```python
from build123d import *

# Parameters (mm, degrees)
F0_R     = 127
F1_DEPTH = 127


with BuildPart() as f1:
    # F0 (on Front) → F1 (new body)
    with BuildSketch(Plane.XZ):
        with BuildLine():
            ThreePointArc((-317.5, 641.227615), (0, 323.727615), (317.5, 641.227615))
            ThreePointArc((317.5, 641.227615), (0, 958.727615), (-317.5, 641.227615))
        make_face()
        with Locations((0, 641.227615)):
            Circle(F0_R, mode=Mode.SUBTRACT)
        with BuildLine():
            Line((317.5, -501.772385), (317.5, 641.227615))
            ThreePointArc((317.5, 641.227615), (0, 323.727615), (-317.5, 641.227615))
            Line((-317.5, 641.227615), (-317.5, -501.772385))
            Line((-317.5, -501.772385), (317.5, -501.772385))
        make_face()
    extrude(amount=F1_DEPTH)


solid = f1.part
```
Design review of the part built by this model. Coordinates are the model's own, in mm. Round coordinates to 2 decimals unless told otherwise and drop trailing zeros. Write each loop counter-clockwise with the first axis right and the second up, starting at its lowest first coordinate (ties: lowest second). Pieces come first, ordered by that corner, then holes. Notation, with made-up numbers: (29.5, 37.25) -> (82.5, 37.25) arc R19 cw to (82.5, 67.25) -> close; hole circle Ø10 at (-20, 8). An arc over 180 degrees is marked (long way). Write item = value, one per line. Start each with the question number.
1) Take a section at B-B, the plane y = -113.5. State the section outline as (x, z) points, plus the area to 3 significant figures.
2) Mouldability with a two-part tool opening along X and no side actions: class faces 1 (the face through (-4, -127, 239)), 2 (the face through (6.98, -62.61, 958.65)), 3 (the face through (-16.533, -62.611, 767.147)) as +X half, -X half, draft (parallel to the pull), parting line (faces both ways), or undercut.
3) Take a section at D-D, the plane x = 153.5. State the section outline as (y, z) points, plus the area to 3 significant figures.
4) Clearance check with a flat-ended pin moving along its axis: pin 1 (1.5 mm diameter, centred on x = 61.5, y = -45, fed in from +Z). State where the tip first meets the part, or that it passes through.
5) Take a section at A-A, the plane x = 0. State the section outline as (y, z) points, plus the area to 3 significant figures.
6) Take a section at C-C, the plane x = 71. State the section outline as (y, z) points, plus the area to 3 significant figures.
7) Wall thickness on probe 1 along Z at (x, y) = (0, -92.5); probe 2 along Z at (x, y) = (-6, -104); probe 3 along X at (y, z) = (-34.5, 566): over which ranges is each line inside the solid? List them lowest first. Write a range as from..to.
Results list:
q1.outline = (-317.5, -501.77) -> (317.5, -501.77) -> (317.5, 641.23) arc R317.5 ccw to (-317.5, 641.23) -> close; hole circle Ø254 at (0, 641.23)
q1.area = 833,000 mm²
q2.face_1 = draft
q2.face_2 = parting line
q2.face_3 = undercut
q3.outline = (-127, -501.77) -> (0, -501.77) -> (0, 919.16) -> (-127, 919.16) -> close
q3.area = 180,000 mm²
q4.pin_1 = 952.86
q5.outline = (-127, -501.77) -> (0, -501.77) -> (0, 514.23) -> (-127, 514.23) -> close; (-127, 768.23) -> (0, 768.23) -> (0, 958.73) -> (-127, 958.73) -> close
q5.area = 153,000 mm²
q6.outline = (-127, -501.77) -> (0, -501.77) -> (0, 535.93) -> (-127, 535.93) -> close; (-127, 746.53) -> (0, 746.53) -> (0, 950.69) -> (-127, 950.69) -> close
q6.area = 158,000 mm²
q7.probe_1 = -501.77..514.23, 768.23..958.73
q7.probe_2 = -501.77..514.37, 768.09..958.67
q7.probe_3 = -317.5..-102.32, 102.32..317.5
